Here's the drawing with two shaded views (mm, measured from the low corner). I have some questions. Give positions to 0.01 mm unless a question says otherwise; leave off trailing zeros. Loops run counter-clockwise (first coordinate to the right, second up) from the corner with the lowest first, then second, coordinate; pieces in that order, holes last. Notation, with made-up numbers: M 1,21 L 50,21 A16 ccw 50,50 Z; hole C 56.5,-2.5 d6. An arc over 180 degrees is marked long. Use CSV: the item, a comma, the result in double quotes.
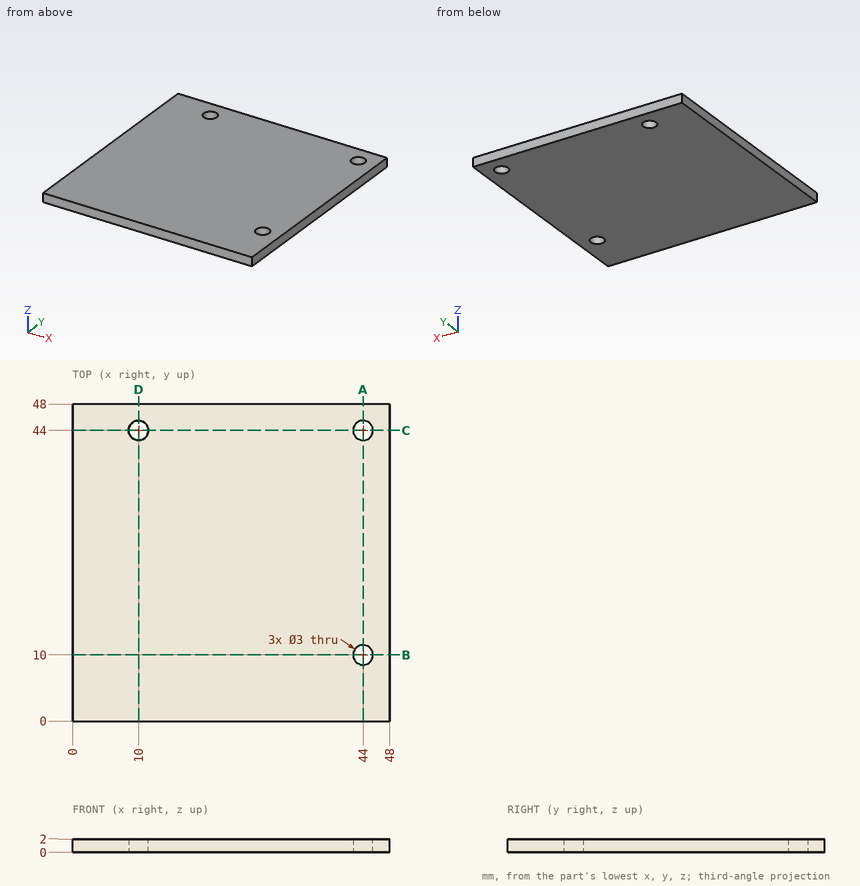
1. I want a section at B-B, the plane y = 10. List the corners of the cut face in (x, z) for me, then the cut area to 3 significant figures.
Outcome:
outline,"M 0,0 L 42.5,0 L 42.5,2 L 0,2 Z; M 45.5,0 L 48,0 L 48,2 L 45.5,2 Z"
area,"90.0 mm2"
2. Please list where these lines run through material, in increasing order: line 1 (Y direction, x = 44, z = 1.45); line 2 (Y direction, x = 10, z = 1.3); line 3 (X direction, y = 44.5, z = 1.55).
Outcome:
line 1,"0 to 8.5, 11.5 to 42.5, 45.5 to 48"
line 2,"0 to 42.5, 45.5 to 48"
line 3,"0 to 8.59, 11.41 to 42.59, 45.41 to 48"
3. I want a section at A-A, the plane x = 44. List the corners of the cut face in (y, z) for me.
Outcome:
outline,"M 0,0 L 8.5,0 L 8.5,2 L 0,2 Z; M 11.5,0 L 42.5,0 L 42.5,2 L 11.5,2 Z; M 45.5,0 L 48,0 L 48,2 L 45.5,2 Z"
